The model under review builds one solid part; all positions refer to its coordinate system, in mm. A direction names the side the tool comes from. Round coordinates to 2 decimals unless told otherwise and drop trailing zeros. Loops run counter-clockwise (first coordinate to the right, second up) from the corner with the lowest first, then second, coordinate; pieces in that order, holes last. Notation, with made-up numbers: (-14, -1.5) -> (40, -1.5) arc R18 ccw to (40, 24.5) -> close; hole circle Ø4 at (73, 89.25). An arc over 180 degrees is marked (long way). Return JSON: item names as keys, results as strings. Group by question number.
```python
from build123d import *

# Parameters (mm, degrees)
BOSS_EXTRUDE1_DEPTH               = 5.5
SKETCH1_3_W                       = 45
SKETCH1_3_H                       = 70
BOSS_EXTRUDE2_DEPTH               = 5.5
TAP_DRILL_FOR_M3_TAP1_D           = 2.5
TAP_DRILL_FOR_M3_TAP1_CSINK_D     = 2.55
TAP_DRILL_FOR_M3_TAP1_CSINK_ANGLE = 90
CHAMFER1_SIZE                     = 2


with BuildPart() as part:
    # Sketch1 → Boss-Extrude1 (new body)
    with BuildSketch(Plane.XY):
        Polygon((-12, -29.5), (22.5, -29.5), (22.5, 40.5), (-22.5, 40.5), (-22.5, -29.5), (-15, -29.5), (-15, -24.5), (-15, 24.5), (15, 24.5), (15, -24.5), (-12, -24.5), align=None)
    extrude(amount=BOSS_EXTRUDE1_DEPTH)

    # Sketch1<3> → Boss-Extrude2 (add)
    with BuildSketch(Plane.XY):
        with Locations((0, 5.5)):
            Rectangle(SKETCH1_3_W, SKETCH1_3_H)
    extrude(amount=-BOSS_EXTRUDE2_DEPTH)

    # Tap Drill for M3 Tap1 (through all)
    with Locations(Plane(origin=(0, 0, -5.5), x_dir=(-1, 0, 0), z_dir=(0, 0, -1))):
        with Locations((20, 38), (-20, 38), (-20, -27), (20, -27)):
            CounterSinkHole(TAP_DRILL_FOR_M3_TAP1_D / 2, TAP_DRILL_FOR_M3_TAP1_CSINK_D / 2, counter_sink_angle=TAP_DRILL_FOR_M3_TAP1_CSINK_ANGLE)

    # Chamfer1
    chamfer1_edges = [part.edges().sort_by_distance(p)[0] for p in [
        (-22.5, -29.5, 0),
        (-22.5, 40.5, 0),
        (22.5, 40.5, 0),
        (22.5, -29.5, 0),
    ]]
    chamfer(chamfer1_edges, length=CHAMFER1_SIZE)


solid = part.part
```
1. Tool access review of faces 1 (the face through (-15, -3, 3)), 2 (the face through (2, -24.5, 3)), 3 (the face through (-21, 40, 0)): name each direction out of +Z, -Z, +X, -X, +Y, -Y from which nothing blocks a thin tool from reaching the whole face with its end or side.
2. We need section B-B, the plane y = 16. Write out the cut boundary in (x, z), then the cut area to 3 significant figures.
3. Draft analysis for pull direction Y (two halves, no side actions). For faces 4 (the face through (21, -29, 0)), 5 (the face through (-18.845, -27.479, 0.089)), 6 (the face through (0, -2, 0)), 7 (the face through (-22.5, 5, 0)), state which applies: pulls with the +Y half, pulls with the -Y half, needs draft (parallel to the pull), parting line crosses it, or undercut.
4. We need section C-C, the plane x = -13.5. Write out the cut boundary in (y, z).
5. We need section A-A, the plane z = 4.25. Write out the cut boundary in (x, y), then the cut area to 3 significant figures.
6. Wall thickness on line 1 (Y direction, x = 20, z = -2.5); line 2 (X direction, y = 38, z = 0.25); line 3 (X direction, y = -11, z = 4.5): over which ranges is each line inside the solid? List them lowest first.
7. We need section D-D, the plane x = 19.5. Give the number of separate pieces and of enclosed holes in the cut face, then the cut area to 3 significant figures.
8. For P1, Ø24, axis at x = -4.5, y = 3, coming from the +Z side; P2, Ø1.5, axis at x = 20, y = -27, coming from the -Z side; P3, Ø8, axis at x = -6.5, y = 15, coming from the +Z side, all flat-tipped, find the tip position at first contact; note any pin that passes through.
Check sheet entries:
{
 "1": {"face 1": "+Z, -Y", "face 2": "+Z", "face 3": "+Z, -Z, -X, +Y"},
 "2": {"outline": "(-22.5, -5.5) -> (22.5, -5.5) -> (22.5, 5.5) -> (15, 5.5) -> (15, 0) -> (-15, 0) -> (-15, 5.5) -> (-22.5, 5.5) -> close", "area": "330 mm²"},
 "3": {"face 4": "pulls with the -Y half", "face 5": "undercut", "face 6": "undercut", "face 7": "needs draft"},
 "4": {"outline": "(-29.5, -5.5) -> (40.5, -5.5) -> (40.5, 5.5) -> (24.5, 5.5) -> (24.5, 0) -> (-29.5, 0) -> close"},
 "5": {"outline": "(-22.5, -27.5) -> (-20.5, -29.5) -> (-15, -29.5) -> (-15, 24.5) -> (15, 24.5) -> (15, -24.5) -> (-12, -24.5) -> (-12, -29.5) -> (20.5, -29.5) -> (22.5, -27.5) -> (22.5, 38.5) -> (20.5, 40.5) -> (-20.5, 40.5) -> (-22.5, 38.5) -> close; hole circle Ø2.5 at (-20, -27); hole circle Ø2.5 at (-20, 38); hole circle Ø2.5 at (20, -27); hole circle Ø2.5 at (20, 38)", "area": "1,640 mm²"},
 "6": {"line 1": "y = -29.5 to -28.25, -25.75 to 36.75, 39.25 to 40.5", "line 2": "x = -22.5 to -21.25, -18.75 to 18.75, 21.25 to 22.5", "line 3": "x = -22.5 to -15, 15 to 22.5"},
 "7": {"separate pieces": "3", "enclosed holes": "0", "area": "720 mm²"},
 "8": {"P1": "stops at z = 5.5", "P2": "passes through", "P3": "stops at z = 0"}
}
